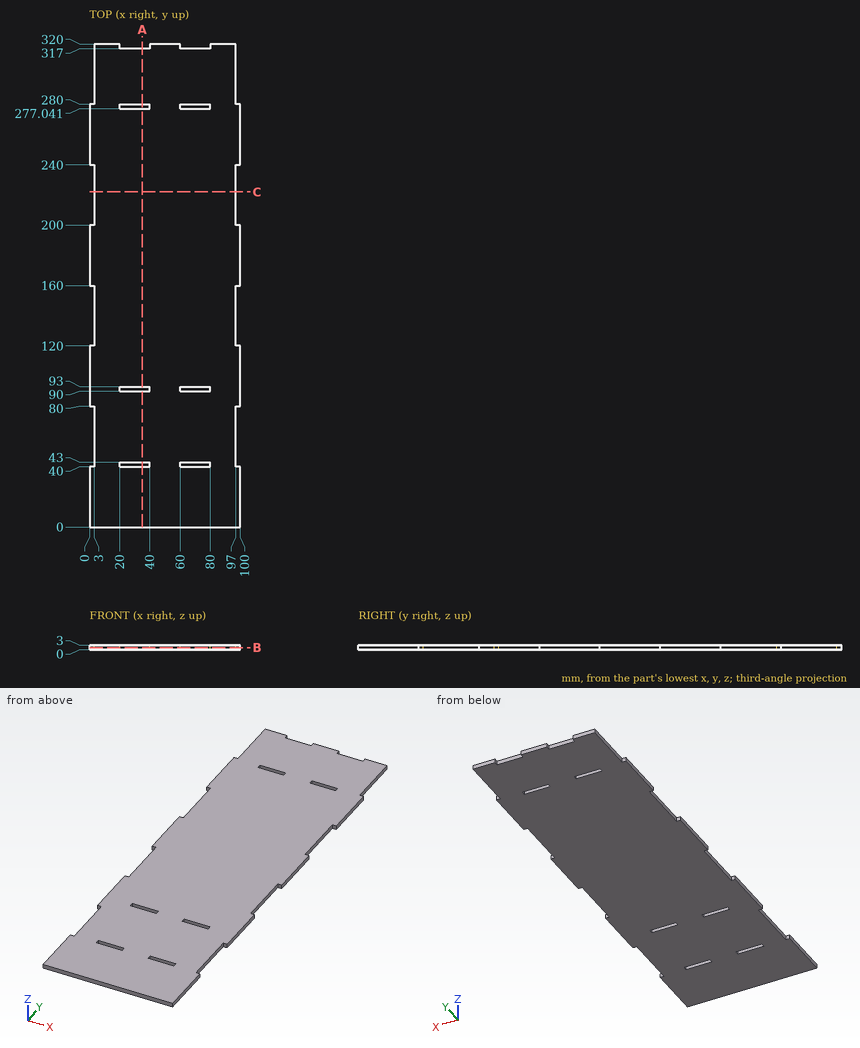
The figure shows three views and two pictorial views of one solid part (mm, origin at its lowest corner). Answer the questions. Give positions to 0.01 mm unless a question says otherwise; leave off trailing zeros. Order: outer loops, then holes, each group sorted by start corner. A loop starts at its lowest first (then second) coordinate and runs counter-clockwise, first axis right, second up. Notation, with made-up numbers: (-17.5, 63) -> (37.5, 63) arc R24 ccw to (37.5, 91) -> close; hole circle Ø3 at (2, -3.75). An arc over 180 degrees is marked (long way). One line per item, written item: value.
1) Find section B-B, the plane z = 1.3. Count the separate pieces of the cut face and the enclosed holes in it, plus the area to 3 significant figures.
Reported:
separate pieces: 1
enclosed holes: 6
area: 30,600 mm^2
2) Find section A-A, the plane x = 35. Determine the outline of the cut face in (y, z).
Reported:
outline: (0, 0) -> (40, 0) -> (40, 3) -> (0, 3) -> close; (43, 0) -> (90, 0) -> (90, 3) -> (43, 3) -> close; (93, 0) -> (277.04, 0) -> (277.04, 3) -> (93, 3) -> close; (280, 0) -> (317, 0) -> (317, 3) -> (280, 3) -> close
3) Find section C-C, the plane y = 222. Determine the outline of the cut face in (x, z), plus the area to 3 significant figures.
Reported:
outline: (3, 0) -> (97, 0) -> (97, 3) -> (3, 3) -> close
area: 282 mm^2
4) Flat-ended cylindrical pins translate along their axes: P1, Ø1.5, axis at x = 34, z = 1.5, coming from the +Y side; P2, Ø1.5, axis at y = 144, z = 1, coming from the -X side; P3, Ø0.9, axis at x = 98, z = 2, coming from the +Y side. Find the tip coordinate at first contact, or state that the pin passes through.
Reported:
P1: stops at y = 317
P2: stops at x = 3
P3: stops at y = 280
5) Find the intervals of material crossed by line 1 (Y direction, x = 20.5, z = 2.85); line 2 (X direction, y = 92.5, z = 0.75); line 3 (X direction, y = 238.5, z = 2.75), in increasing order.
Reported:
line 1: y = 0 to 40, 43 to 90, 93 to 277.04, 280 to 317
line 2: x = 0 to 20, 40 to 60, 80 to 100
line 3: x = 3 to 97
